Build history of the part. All positions in model axes, mm. A direction names the side the tool comes from. Coordinates: 2 decimals unless noted, no trailing zeros. Order: outer loops, then holes, each group sorted by start corner. A loop starts at its lowest first (then second) coordinate and runs counter-clockwise, first axis right, second up. Notation, with made-up numbers: (-12.75, 51) - (11.25, 51) arc R20 ccw to (11.25, 63) - close; hole circle Ø2 at (24, 58.25). An arc over 180 degrees is marked (long way). Return JSON: item names as keys, results as strings.
Autodesk Fusion 360 part; units mm, degrees
sketch "base" plane through (0, 0, 0) normal (0, 1, 0) x (1, 0, 0)
  line L0 (36.5, -32.9) -> (-36.5, -32.9)
  line L1 (-36.5, -32.9) -> (-36.5, -30.9)
  line L2 (-36.5, -30.9) -> (36.5, -30.9)
  line L3 (36.5, -30.9) -> (36.5, -32.9)
  line L4 (36.5, 32.9) -> (-36.5, 32.9)
  line L5 (-36.5, 32.9) -> (-36.5, 30.9)
  line L6 (-36.5, 30.9) -> (36.5, 30.9)
  line L7 (36.5, 30.9) -> (36.5, 32.9)
  line L8 (36.5, -30.9) -> (34.5, -30.9)
  line L9 (34.5, -30.9) -> (34.5, 30.9)
  line L10 (34.5, 30.9) -> (36.5, 30.9)
  line L11 (36.5, 30.9) -> (36.5, -30.9)
  line L12 (0, -49.6148) -> (0, 45.2004) construction
  line L13 (54.9351, 0) -> (-34.717, 0) construction
  line L14 (-36.5, -30.9) -> (-34.5, -30.9)
  line L15 (-34.5, -30.9) -> (-34.5, 30.9)
  line L16 (-34.5, 30.9) -> (-36.5, 30.9)
  line L17 (-36.5, 30.9) -> (-36.5, -30.9)
  dimension "d1" = 2
  dimension "d2" = 73
  dimension "d3" = 65.8
extrude "Extrude1" add sketch "base" along normal blind 55 contours L0 L1 L2 L3 L8 L14 | L2 L6 L8 L9 L10 L11 | L2 L6 L14 L15 L16 L17 | L4 L5 L6 L7 L10 L16 makes body 1
extrude "Extrude2" add sketch "base" along normal blind 4 separate body contours L2 L6 L9 L15 makes body 2
sketch "Sketch3" plane through (0, 4, 0) normal (0, 1, 0) x (-1, 0, 0)
  line L0 (-34.5, 30.9) -> (-34.5, -30.9)
  line L1 (-34.5, -30.9) -> (34.5, -30.9)
  line L2 (34.5, -30.9) -> (34.5, 30.9)
  line L3 (34.5, 30.9) -> (-34.5, 30.9)
  line L4 (-32.5, -28.9) -> (32.5, -28.9)
  line L5 (32.5, -28.9) -> (32.5, 28.9)
  line L6 (32.5, 28.9) -> (-32.5, 28.9)
  line L7 (-32.5, 28.9) -> (-32.5, -28.9)
  dimension "d16" = -2
extrude "Extrude5" add sketch "Sketch3" along normal blind 47.2 bodies 1 2
equation "d17 = 56 mm - 3.8 mm - 5 mm"
1. Probe L1, parallel to X at y = 23, z = -0.5; L2, parallel to Z at x = 13, y = 50.5; L3, parallel to Y at x = 19.5, z = -17.5. List the from-to ranges inside material, lowest first.
Check values:
{"L1": "-36.5 to -32.5, 32.5 to 36.5", "L2": "-32.9 to -28.9, 28.9 to 32.9", "L3": "0 to 4"}
2. Drop a flat-ended pin along its axis: pin 1 (5 mm diameter, centred on x = 22, z = -2, fed in from +Y). Give the stop position or say it passes through.
Check values:
{"pin 1": "y = 4"}
3. Cut at A-A on y = 42.5. Give the cut face in (x, z).
Check values:
{"outline": "(-36.5, -32.9) - (36.5, -32.9) - (36.5, 32.9) - (-36.5, 32.9) - close; hole (-32.5, -28.9) - (32.5, -28.9) - (32.5, 28.9) - (-32.5, 28.9) - close"}
4. Mould opens along X. For faces 1 (the flat face through (1, 27, 32.9)), 2 (the flat face through (34.5, 53, 0)), 3 (the flat face through (-36.5, 27, 0)) say: pulls with the +X half, pulls with the -X half, needs draft (parallel to the pull), parting line crosses it, or undercut.
Check values:
{"face 1": "needs draft", "face 2": "undercut", "face 3": "pulls with the -X half"}
5. Cut at C-C on x = -23.5. Give the cut face in (y, z).
Check values:
{"outline": "(0, -32.9) - (55, -32.9) - (55, -30.9) - (51.2, -30.9) - (51.2, -28.9) - (4, -28.9) - (4, 28.9) - (51.2, 28.9) - (51.2, 30.9) - (55, 30.9) - (55, 32.9) - (0, 32.9) - close"}
6. Tool access for faces 4 (the flat face through (0, 53, 30.9)), 5 (the flat face through (-1, 0, 0)): list every direction of +Z, -Z, +X, -X, +Y, -Y with a clear straight run to the whole face (end or side of a thin tool).
Check values:
{"face 4": "+Y", "face 5": "+Z, -Z, +X, -X, -Y"}
7. Cut at B-B on z = -22. Give the cut face in (x, y).
Check values:
{"outline": "(-36.5, 0) - (36.5, 0) - (36.5, 55) - (34.5, 55) - (34.5, 51.2) - (32.5, 51.2) - (32.5, 4) - (-32.5, 4) - (-32.5, 51.2) - (-34.5, 51.2) - (-34.5, 55) - (-36.5, 55) - close"}
